The model under review builds one solid part; all positions refer to its coordinate system, in mm. Coordinates: 2 decimals unless noted, no trailing zeros. Write each loop counter-clockwise with the first axis right and the second up, starting at its lowest first coordinate (ties: lowest second). Pieces come first, ordered by that corner, then holes. Notation, with made-up numbers: (44, -17) - (76, -17) arc R22 cw to (76, -8) - close; hole circle Ø10 at (84, -35.5). An arc over 180 degrees is marked (long way). Return JSON: item names as keys, results as strings. Group by question number.
(1) We need section A-A on x = 22.5. State the section outline as (y, z) points.
(2) For pin 1 Ø0.9 at (y, z) = (-29.5, 0.5) entering from +X; pin 2 Ø20 at (x, y) = (20.5, -57.5) entering from +Z; pin 3 Ø0.9 at (y, z) = (31, 0.5) entering from -X, all flat-tipped, find the tip position at first contact; note any pin that passes through.
(3) We need section B-B on x = -27.5. State the section outline as (y, z) points.
(4) To check wall thickness, follow L1, parallel to Y at x = 21, z = -0.8; L2, parallel to Y at x = -26.5, z = -1.2; L3, parallel to X at y = 33, z = -1.1. State the ranges of each line that lie inside material, in increasing order. Write a range as from..to.
```python
from build123d import *

# Parameters (mm, degrees)
F0_R     = 12.5
F1_DEPTH = 1.5


# Not quite as in the source:
# - ends of sketch curves that miss each other by under 0.0002 mm in the source are joined


with BuildPart() as f1:
    # F0 (on Top) → F1 (new body, symmetric)
    with BuildSketch(Plane.XY):
        Polygon((-46.9999983907, 3.8743e-06), (-46.9999983907, -4.9999961257), (-43.9999983907, -4.9999961257), (-43.9999983907, -14.9999961257), (-46.9999983907, -14.9999961257), (-46.9999983907, -24.9999961257), (-43.9999983907, -24.9999961257), (-43.9999983907, -34.9999961257), (-46.9999983907, -34.9999961257), (-46.9999983907, -44.9999961257), (-43.9999983907, -44.9999961257), (-43.9999983907, -54.9999961257), (-46.9999983907, -54.9999961257), (-46.9999983907, -64.9999961257), (-43.9999983907, -64.9999961257), (-43.9999983907, -74.9999961257), (-46.9999983907, -74.9999961257), (-46.9999983907, -89.9999961257), (-31.9999983907, -89.9999961257), (-31.9999983907, -86.9999961257), (-21.9999983907, -86.9999961257), (-21.9999983907, -89.9999961257), (-11.9999983907, -89.9999961257), (-11.9999983907, -86.9999961257), (-1.9999983907, -86.9999961257), (-1.9999983907, -89.9999961257), (8.0000016093, -89.9999961257), (8.0000016093, -86.9999961257), (18.0000016093, -86.9999961257), (18.0000016093, -89.9999961257), (28.0000016093, -89.9999961257), (28.0000016093, -86.9999961257), (38.0000016093, -86.9999961257), (38.0000016093, -89.9999961257), (53.0000016093, -89.9999961257), (53.0000030994, -75.968132019), (50.0000030994, -75.968132019), (50.0000030994, -65.968132019), (53.0000030994, -65.968132019), (53.0000030994, -55.968132019), (50.0000030994, -55.968132019), (50.0000030994, -45.968132019), (53.0000030994, -45.968132019), (53.0000030994, -35.968132019), (50.0000030994, -35.968132019), (50.0000030994, -25.968132019), (53.0000030994, -25.968132019), (53.0000030994, -15.968132019), (50.0000030994, -15.968132019), (50.0000030994, -5.968132019), (53.0000030994, -5.968132019), (53.0000030994, 3.8743e-06), (53.0000030994, 4.031867981), (50.0000030994, 4.031867981), (50.0000030994, 14.031867981), (53.0000030994, 14.031867981), (53.0000030994, 24.031867981), (50.0000030994, 24.031867981), (50.0000030994, 34.031867981), (53.0000030994, 34.031867981), (53.0000030994, 44.031867981), (50.0000030994, 44.031867981), (50.0000030994, 54.031867981), (53.0000030994, 54.031867981), (53.0000030994, 64.031867981), (50.0000030994, 64.031867981), (50.0000030994, 74.031867981), (53.0000030994, 74.031867981), (53.0000030994, 90.0000038743), (38.0000016093, 90.0000035763), (38.0000016093, 87.0000035763), (28.0000016093, 87.0000035763), (28.0000016093, 90.0000035763), (18.0000016093, 90.0000035763), (18.0000016093, 87.0000035763), (8.0000016093, 87.0000035763), (8.0000016093, 90.0000035763), (-1.9999983907, 90.0000035763), (-1.9999983907, 87.0000035763), (-11.9999983907, 87.0000035763), (-11.9999983907, 90.0000035763), (-21.9999983907, 90.0000035763), (-21.9999983907, 87.0000035763), (-31.9999983907, 87.0000035763), (-31.9999983907, 90.0000035763), (-46.9999983907, 90.0000035763), (-46.9999983907, 75.0000038743), (-43.9999983907, 75.0000038743), (-43.9999983907, 65.0000038743), (-46.9999983907, 65.0000038743), (-46.9999983907, 55.0000038743), (-43.9999983907, 55.0000038743), (-43.9999983907, 45.0000038743), (-46.9999983907, 45.0000038743), (-46.9999983907, 35.0000038743), (-43.9999983907, 35.0000038743), (-43.9999983907, 25.0000038743), (-46.9999983907, 25.0000038743), (-46.9999983907, 15.0000038743), (-43.9999983907, 15.0000038743), (-43.9999983907, 5.0000038743), (-46.9999983907, 5.0000038743), align=None)
        with Locations((20.5000030994, -57.4999969183)):
            Circle(F0_R, mode=Mode.SUBTRACT)
    extrude(amount=F1_DEPTH, both=True)


solid = f1.part
```
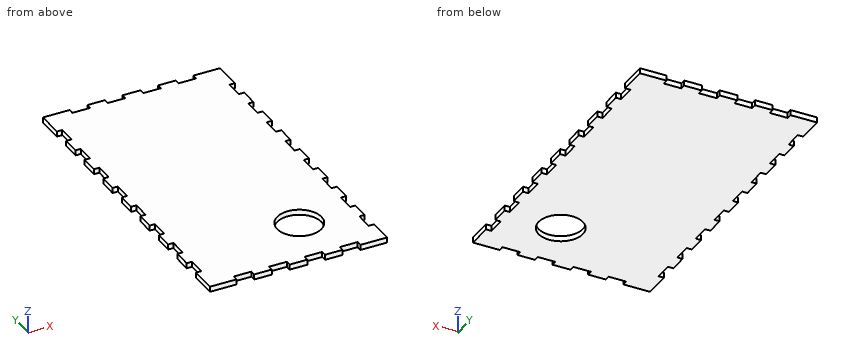
Ans:
{
 "1": {"outline": "(-90, -1.5) - (-69.84, -1.5) - (-69.84, 1.5) - (-90, 1.5) - close; (-45.16, -1.5) - (90, -1.5) - (90, 1.5) - (-45.16, 1.5) - close"},
 "2": {"pin 1": "x = 50", "pin 2": "through", "pin 3": "x = -44"},
 "3": {"outline": "(-87, -1.5) - (87, -1.5) - (87, 1.5) - (-87, 1.5) - close"},
 "4": {"L1": "-90..-69.99, -45.01..90", "L2": "-87..87", "L3": "-44..50"}
}
